Read the model definition and answer for the solid it produces. Units are mm, in the model's axes. A direction names the side the tool comes from. Round coordinates to 2 decimals unless told otherwise and drop trailing zeros. Write each loop counter-clockwise with the first axis right and the second up, starting at its lowest first coordinate (ties: lowest second). Pieces come first, ordered by that corner, then holes. Notation, with made-up numbers: (13.25, -1) -> (19.25, -1) arc R27 cw to (19.25, 32) -> close; hole circle Ø10 at (32.5, -23). An arc over 180 degrees is marked (long way). Return JSON: item names as keys, results as strings. Group by question number.
(1) For faces 4 (the conical face through (0.173, 11.133, 0.135)), 5 (the flat face through (0, 3, 9)), determine the directions among +Z, -Z, +X, -X, +Y, -Y from which every point of the face is accessible in a straight line to the end or side of a thin tool.
(2) The mould has two halves that part along X. Classify faces 1 (the flat face through (0, 7, 6)), 2 (the cylindrical face through (0.18, 11.5, 5.27)), 3 (the flat face through (0, 5, 0)): released by +X, released by -X, zero draft, split by the parting line, or undercut.
(3) Given pin 1 (5.5 mm diameter, centred on y = 5, z = 11, fed in from +X); pin 2 (4 mm diameter, centred on y = 7, z = 9.5, fed in from +X); pin 3 (3 mm diameter, centred on x = 6, z = 6.5, fed in from +Y); pin 4 (0.6 mm diameter, centred on x = 0.5, z = 13, fed in from +Y), each flat-ended and moving along its own axis, determine where each tip first touches the part or whether it passes through.
(4) Straight lines are drawn through the part: line 1 (Z direction, x = -0.25, y = 5.75); line 2 (X direction, y = 5.75, z = 9.5); line 3 (X direction, y = 9.25, z = 11.5). For each, find the intervals that lie inside material, in ascending order.
(5) A cutting plane is placed at B-B on z = 9.5. Give the vertices of the cut face in (x, y).
```python
from build123d import *

# Parameters (mm, degrees)
F4_DEPTH  = 1
F6_DEPTH  = 12
F7_SIZE   = 0.5
F8_W      = 6
F8_H      = 3
F9_DEPTH  = 12
F10_DEPTH = 5
F11_W     = 6
F11_H     = 1.5
F12_DEPTH = 1
F13_SIZE  = 0.99999


# Not quite as in the source:
# - a fillet or chamfer is up to 0.001 mm smaller than in the source, because OpenCascade refuses the exact size


with BuildPart() as f4:
    # F3 (on Top) → F4 (new body)
    with BuildSketch(Plane.XY):
        with BuildLine():
            Line((-8.25, 0), (0, 0))
            Line((0, 0), (8.25, 0))
            Line((8.25, 0), (8.25, 3.25))
            ThreePointArc((8.25, 3.25), (0, 11.5), (-8.25, 3.25))
            Line((-8.25, 3.25), (-8.25, 0))
        make_face()
    extrude(amount=F4_DEPTH)

    # F5 (on face) → F6 (join)
    with BuildSketch(Plane.XY.offset(1)):
        with BuildLine():
            Line((-3, 0), (-3, 10.9352130745))
            ThreePointArc((-3, 10.9352130745), (-6.8122132967, 7.9036276172), (-8.25, 3.25))
            Line((-8.25, 3.25), (-8.25, 0))
            Line((-8.25, 0), (-3, 0))
        make_face()
        with BuildLine():
            ThreePointArc((8.25, 3.25), (6.8122132967, 7.9036276172), (3, 10.9352130745))
            Line((3, 10.9352130745), (3, 0))
            Line((3, 0), (8.25, 0))
            Line((8.25, 0), (8.25, 3.25))
        make_face()
    extrude(amount=F6_DEPTH)

    # F7
    f7_edges = [f4.edges().sort_by_distance(p)[0] for p in [
        (8.25, 1.625, 0),
        (0, 0, 0),
    ]]
    chamfer(f7_edges, length=F7_SIZE)

    # F8 (on face) → F9 (join)
    with BuildSketch(Plane.XY.offset(1)):
        with Locations((0, 1.5)):
            Rectangle(F8_W, F8_H)
    extrude(amount=F9_DEPTH)

    # F10 (add): a face of the model
    f10_faces = [f4.faces().sort_by_distance(p)[0] for p in [
        (0, 7.1588841066, 1),
    ]]
    extrude(f10_faces, amount=F10_DEPTH)

    # F11 (on face) → F12 (join)
    with BuildSketch(Plane(origin=(0, 3, 0), x_dir=(-1, 0, 0), z_dir=(0, 1, 0))):
        with Locations((0, 12.25)):
            Rectangle(F11_W, F11_H)
    extrude(amount=F12_DEPTH)

    # F13 (size 1 in the source; OpenCascade refuses exactly that, so slightly less here)
    f13_edges = [f4.edges().sort_by_distance(p)[0] for p in [
        (0, 4, 11.5),
    ]]
    chamfer(f13_edges, length=F13_SIZE)


solid = f4.part
```
Checks:
{
 "1": {"face 4": "-Z, +Y", "face 5": "+Y"},
 "2": {"face 1": "undercut", "face 2": "split by the parting line", "face 3": "zero draft"},
 "3": {"pin 1": "stops at x = 8.25", "pin 2": "stops at x = 8.06", "pin 3": "stops at y = 10.16", "pin 4": "stops at y = 4"},
 "4": {"line 1": "z = 0 to 6", "line 2": "x = -7.86 to -3, 3 to 7.86", "line 3": "x = -5.66 to -3, 3 to 5.66"},
 "5": {"outline": "(-8.25, 0) -> (8.25, 0) -> (8.25, 3.25) arc R8.25 ccw to (3, 10.94) -> (3, 3) -> (-3, 3) -> (-3, 10.94) arc R8.25 ccw to (-8.25, 3.25) -> close"}
}
